Study the drawing (mm; zero at the part's minimum x, y, z) and answer. A direction names the side the tool comes from. Round coordinates to 2 decimals unless told otherwise and drop trailing zeros. Write each loop counter-clockwise with the first axis right and the second up, starting at its lowest first coordinate (ties: lowest second). Pieces come first, ordered by that corner, then holes. Notation, with made-up numbers: (-2, 13) -> (53, 13) arc R16 cw to (53, 24) -> close; hole circle Ø3 at (29, 14.5). An arc over 180 degrees is marked (long way). Return JSON: item names as keys, results as strings.
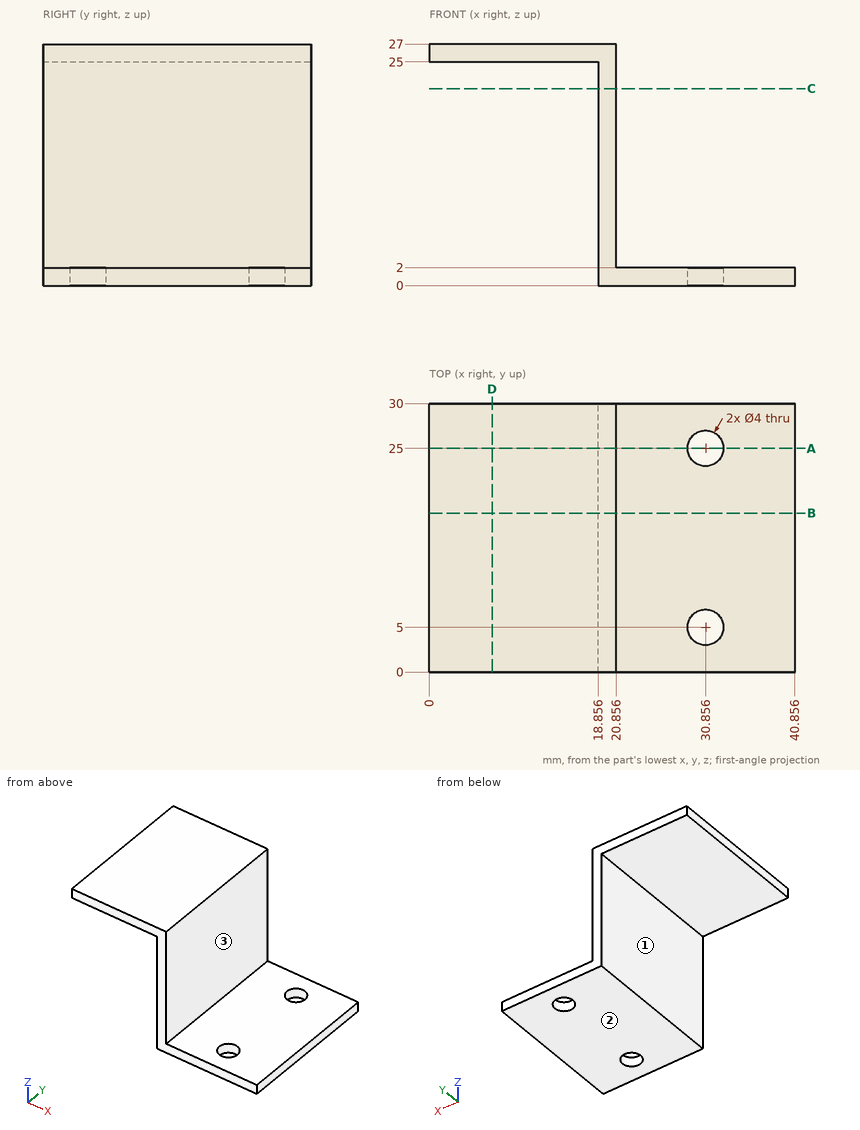
Item 1: Section C-C (z = 22) is taken. Give the vertices of the cut face in (x, y), then the cut area to 3 significant figures.
Worked answers:
{"outline": "(18.86, 0) -> (20.86, 0) -> (20.86, 30) -> (18.86, 30) -> close", "area": "60.0 mm2"}
Item 2: Flat-ended cylindrical pins translate along their axes: pin 1 (5 mm diameter, centred on x = 30.86, y = 5, fed in from +Z); pin 2 (15 mm diameter, centred on x = 9, y = 8.5, fed in from -Z); pin 3 (4 mm diameter, centred on y = 22.5, z = 14.5, fed in from +X). Find the tip coordinate at first contact, or state that the pin passes through.
Worked answers:
{"pin 1": "stops at z = 2", "pin 2": "stops at z = 25", "pin 3": "stops at x = 20.86"}
Item 3: Section A-A (y = 25) is taken. Give the vertices of the cut face in (x, z), then the cut area to 3 significant figures.
Worked answers:
{"outline": "(0, 25) -> (18.86, 25) -> (18.86, 0) -> (28.86, 0) -> (28.86, 2) -> (20.86, 2) -> (20.86, 27) -> (0, 27) -> close; (32.86, 0) -> (40.86, 0) -> (40.86, 2) -> (32.86, 2) -> close", "area": "124 mm2"}
Item 4: Section D-D (x = 7) is taken. Give the vertices of the cut face in (y, z).
Worked answers:
{"outline": "(0, 25) -> (30, 25) -> (30, 27) -> (0, 27) -> close"}
Item 5: A tool of negligible diameter and unlimited length cuts with its end or side. For the marked faces 1, 2 and 3, from which of +Z, -Z, +X, -X, +Y, -Y can it reach the whole face along a straight path? Write none if from no direction.
Worked answers:
{"face 1": "-Z, -X, +Y, -Y", "face 2": "-Z, +X, -X, +Y, -Y", "face 3": "+Z, +X, +Y, -Y"}
Item 6: Section B-B (y = 17.75) is taken. Give the vertices of the cut face in (x, z), then the cut area to 3 significant figures.
Worked answers:
{"outline": "(0, 25) -> (18.86, 25) -> (18.86, 0) -> (40.86, 0) -> (40.86, 2) -> (20.86, 2) -> (20.86, 27) -> (0, 27) -> close", "area": "132 mm2"}
Item 7: Straight lines are drawn through the part: L1, parallel to X at y = 13, z = 25.25; L2, parallel to X at y = 22.25, z = 23; L3, parallel to Z at x = 36, y = 14. For each, find the intervals that lie inside material, in ascending order. Write a range as [from, to].
Worked answers:
{"L1": "x = [0, 20.86]", "L2": "x = [18.86, 20.86]", "L3": "z = [0, 2]"}
